```python
from build123d import *

# Parameters (mm, degrees)
F0_W     = 38.1
F0_H     = 38.1
F1_DEPTH = 0.79375
F2_W     = 38.1
F2_H     = 38.1
F2_W_2   = 34.925
F2_H_2   = 34.925
F3_DEPTH = 1.5875
F4_W     = 1.27
F4_H     = 30.4073842667
F4_W_2   = 7.8308774173
F4_H_2   = 1.5500376467
F4_W_3   = 4.9481987953
F4_H_3   = 6.1405338347
F4_W_4   = 7.175091283
F4_H_4   = 2.9808413237
F4_W_5   = 1.311570406
F4_H_5   = 7.3952877388
F5_DEPTH = 1.5875
F6_R     = 1.27
F7_DEPTH = 0.396875


with BuildPart() as f1:
    # F0 (on Top) → F1 (new body)
    with BuildSketch(Plane.XY):
        with Locations((2.9509142041, -6.7803348825)):
            Rectangle(F0_W, F0_H)
    extrude(amount=F1_DEPTH)

    # F2 (on face) → F3 (join)
    with BuildSketch(Plane.XY.offset(0.79375)):
        with Locations((2.9509142041, -6.7803348825)):
            Rectangle(F2_W, F2_H)
        with Locations((2.9509142041, -6.7803348825)):
            Rectangle(F2_W_2, F2_H_2, mode=Mode.SUBTRACT)
    extrude(amount=F3_DEPTH)

    # F4 (on face) → F5 (join)
    with BuildSketch(Plane.XY.offset(0.79375)):
        with Locations((-9.3176252598, -9.0391427491)):
            Rectangle(F4_W, F4_H)
        Polygon((9.5420787111, 6.1645493843), (-3.6026252598, 6.1645493843), (-3.6026252598, 4.9125957303), (8.3497418091, 4.9125957303), (8.3497418091, 1.6336699482), (-6.0775312595, 1.6336699482), (-6.0775312595, 0.3220996878), (8.3497418091, 0.3220996878), (8.3497418091, -11.6012664512), (3.0736522749, -11.6012664512), (3.0736522749, -3.4337604884), (1.5534231206, -3.4337604884), (1.5534231206, -11.6012664512), (-2.2024372593, -11.6012664512), (-2.2024372593, -12.8532201052), (8.3497418091, -12.8532201052), (9.5420787111, -12.8532201052), (9.5420787111, 3.1240906101), (17.113417387, 3.1240906101), (17.113417387, 4.9125957303), (9.5420787111, 4.9125957303), align=None)
        with Locations((16.4979754955, -2.6587416651)):
            Rectangle(F4_W_2, F4_H_2)
        with Locations((15.0566361845, -10.5579718947)):
            Rectangle(F4_W_3, F4_H_3)
        with Locations((16.8258685626, -19.5303047076)):
            Rectangle(F4_W_4, F4_H_4)
        with Locations((10.1978639141, -20.5451910131)):
            Rectangle(F4_W_5, F4_H_5)
        Polygon((-4.8255776055, -15.2975097299), (-4.8255776055, -24.2428348825), (-3.5736244172, -24.2428348825), (-3.5736244172, -16.8475471437), (5.8458349667, -16.8475471437), (5.8458349667, -24.2428348825), (7.0977881551, -24.2428348825), (7.0977881551, -15.2975097299), align=None)
    extrude(amount=F5_DEPTH)

    # F6 (on face) → F7 (cut)
    with BuildSketch(Plane.XY.offset(0.79375)):
        with Locations((-12.2321055278, -20.8758749068)):
            Circle(F6_R)
        with Locations((18.6622906476, -22.631780126)):
            Circle(F6_R)
    extrude(amount=-F7_DEPTH, mode=Mode.SUBTRACT)


solid = f1.part
```
Model file for the job. Use its own axes, mm. A direction names the side the tool comes from. Give positions to 0.01 mm unless a question says otherwise; leave off trailing zeros. Loops run counter-clockwise (first coordinate to the right, second up) from the corner with the lowest first, then second, coordinate; pieces in that order, holes last. Notation, with made-up numbers: (15.5, 6.25) - (59.5, 6.25) arc R16 cw to (59.5, 23.25) - close; hole circle Ø4 at (18, -29.75). An arc over 180 degrees is marked (long way). One line per item, written item: value. Start each with the question number.
1. Slice it at B-B (x = 10). List the corners of the cut face in (y, z), plus the area to 3 significant figures.
2. Pull direction Y, two halves, no side cores. Call faces 3 (the cylindrical face through (-12.507, -22.116, 0.598)), 4 (the flat face through (1, -24.243, 2)), 5 (the flat face through (-16.099, -7, 1)): pulls with the +Y half, pulls with the -Y half, needs draft (parallel to the pull), parting line crosses it, or undercut.
3. Which spindle directions (+Z, -Z, +X, -X, +Y, -Y) get a long thin tool onto all of the face, cutting with end or side? Do faces 1 (the flat face through (1.5, -16.6, 2.381)), 2 (the flat face through (16, -24.243, 2)). Say none if no direction does.
4. Pin check, flat tip, straight feed: pin 1 (1.5 mm diameter, centred on x = -12.23, y = -20.88, fed in from +Z). Stop position of the tip, or through.
5. Slice it at A-A (y = 7). List the corners of the cut face in (x, z).
6. Probe L1, parallel to X at y = -5, z = 1.9; L2, parallel to X at y = 4.5, z = 1.45; L3, parallel to X at y = 2, z = 1.2. List the from-to ranges inside material, lowest first. Write a range as from..to.
7. Slice it at D-D (x = -8). List the corners of the cut face in (y, z).
8. Slice it at C-C (z = 1.75). Give the number of separate pieces and of enclosed holes in the cut face, plus the area to 3 significant figures.
Solution:
1. outline: (-25.83, 0) - (12.27, 0) - (12.27, 2.38) - (10.68, 2.38) - (10.68, 0.79) - (4.91, 0.79) - (4.91, 2.38) - (3.12, 2.38) - (3.12, 0.79) - (-16.85, 0.79) - (-16.85, 2.38) - (-25.83, 2.38) - close
1. area: 49.9 mm^2
2. face 3: undercut
2. face 4: undercut
2. face 5: needs draft
3. face 1: +Z, +X, -X, +Y, -Y
3. face 2: +Z
4. pin 1: stops at z = 0.4
5. outline: (-16.1, 0) - (22, 0) - (22, 2.38) - (20.41, 2.38) - (20.41, 0.79) - (-14.51, 0.79) - (-14.51, 2.38) - (-16.1, 2.38) - close
6. L1: x = -16.1..-14.51, -9.95..-8.68, 1.55..3.07, 8.35..9.54, 20.41..22
6. L2: x = -16.1..-14.51, -9.95..-8.68, 8.35..17.11, 20.41..22
6. L3: x = -16.1..-14.51, -9.95..-8.68, 8.35..9.54, 20.41..22
7. outline: (-25.83, 0) - (12.27, 0) - (12.27, 2.38) - (10.68, 2.38) - (10.68, 0.79) - (-24.24, 0.79) - (-24.24, 2.38) - (-25.83, 2.38) - close
8. separate pieces: 3
8. enclosed holes: 2
8. area: 477 mm^2
